Input: part model. Units: mm. Frame: model coordinates. Face numbers are marked on the shaded views. A direction names the side the tool comes from. Give positions to 0.01 mm unless a question says otherwise; leave off trailing zeros. Loops run counter-clockwise (first coordinate to the right, second up) from the corner with the lowest first, then second, coordinate; pieces in that order, holes last.
from build123d import *

# Parameters (mm, degrees)
F0_W     = 45
F0_H     = 44
F1_DEPTH = 23
F2_W     = 5
F2_H     = 5
F3_DEPTH = 5
F5_W     = 59
F5_H     = 23
F6_DEPTH = 2.75
F7_R     = 1


with BuildPart() as f1:
    # F0 (on Front) → F1 (new body)
    with BuildSketch(Plane.XZ):
        with Locations((22.5, 22)):
            Rectangle(F0_W, F0_H)
    extrude(amount=F1_DEPTH)

    # F2 (on face) → F3 (join)
    with BuildSketch(Plane.XY.offset(44)):
        with Locations((33, -11.5)):
            Rectangle(F2_W, F2_H)
    extrude(amount=F3_DEPTH)

    # F5 (on offset) → F6 (join)
    with BuildSketch(Plane.XY.offset(30)):
        with Locations((22.5, -11.5)):
            Rectangle(F5_W, F5_H)
    extrude(amount=F6_DEPTH)

    # F7
    f7_edges = [f1.edges().sort_by_distance(p)[0] for p in [
        (45, -11.5, 44),
        (22.5, 0, 44),
        (22.5, -23, 44),
        (0, -11.5, 44),
        (33, -9, 44),
        (35.5, -11.5, 44),
        (33, -14, 44),
        (30.5, -11.5, 44),
        (0, -11.5, 0),
        (45, -11.5, 0),
        (22.5, 0, 0),
        (22.5, -23, 0),
        (45, -23, 15),
        (45, 0, 15),
        (0, -23, 15),
        (0, -23, 38.375),
        (45, -23, 38.375),
        (45, 0, 38.375),
        (0, 0, 38.375),
        (0, 0, 15),
    ]]
    fillet(f7_edges, radius=F7_R)


solid = f1.part
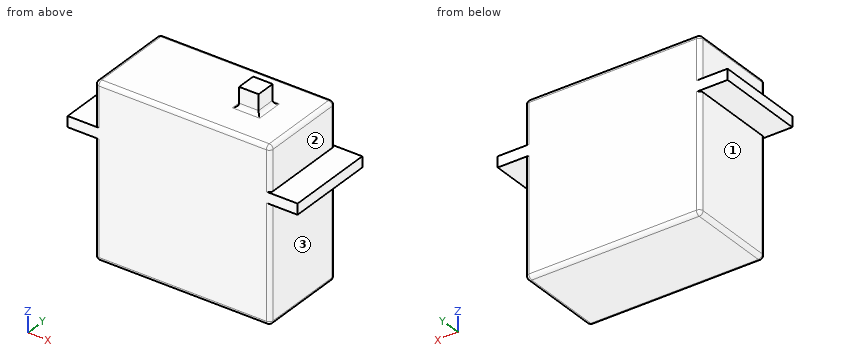
(1) Pin query (flat end, axial travel): pin 1 Ø4 at (x, y) = (-1.5, -12.5) entering from -Z; pin 2 Ø1.5 at (x, y) = (5, -20) entering from +Z; pin 3 Ø10 at (y, z) = (-4.5, 16.5) entering from -X. Return the tip coordinate at first contact, or that it passes through.
Values follow:
pin 1: stops at z = 0.13
pin 2: stops at z = 44
pin 3: stops at x = 0
(2) Cut plane B-B (x = 10). Return the cut outline in (y, z).
Values follow:
outline: (-23, 1) arc R1 ccw to (-22, 0) - (-1, 0) arc R1 ccw to (0, 1) - (0, 43) arc R1 ccw to (-1, 44) - (-22, 44) arc R1 ccw to (-23, 43) - close
(3) Ray query, probe 1 along Z at (x, y) = (24, -4.25); probe 2 along X at (y, z) = (-15.5, 37.5); probe 3 along Z at (x, y) = (47, -10.75). Return the intervals inside material, ascending.
Values follow:
probe 1: z = 0 to 44
probe 2: x = 0 to 45
probe 3: z = 30 to 32.75
(4) Reachability of the marked faces 1, 2 and 3 from +Z, -Z, +X, -X, +Y, -Y: full face, straight path, thin tool, end or side. Return the list, or none.
Values follow:
face 1: -Z, -X, +Y, -Y
face 2: +Z, +X, +Y, -Y
face 3: -Z, +X, +Y, -Y
(5) Cut plane D-D (y = -11.5). Return the cut outline in (x, z).
Values follow:
outline: (-7, 30) - (0, 30) - (0, 1) arc R1 ccw to (1, 0) - (44, 0) arc R1 ccw to (45, 1) - (45, 30) - (52, 30) - (52, 32.75) - (45, 32.75) - (45, 43) arc R1 ccw to (44, 44) - (36.5, 44) arc R1 cw to (35.5, 45) - (35.5, 49) - (30.5, 49) - (30.5, 45) arc R1 cw to (29.5, 44) - (1, 44) arc R1 ccw to (0, 43) - (0, 32.75) - (-7, 32.75) - close
(6) Cut plane A-A (z = 15). Return the cut outline in (x, y).
Values follow:
outline: (0, -22) arc R1 ccw to (1, -23) - (44, -23) arc R1 ccw to (45, -22) - (45, -1) arc R1 ccw to (44, 0) - (1, 0) arc R1 ccw to (0, -1) - close
(7) Cut plane C-C (y = -4.5). Return the cut outline in (x, z), and give its area (3 significant figures).
Values follow:
outline: (-7, 30) - (0, 30) - (0, 1) arc R1 ccw to (1, 0) - (44, 0) arc R1 ccw to (45, 1) - (45, 30) - (52, 30) - (52, 32.75) - (45, 32.75) - (45, 43) arc R1 ccw to (44, 44) - (1, 44) arc R1 ccw to (0, 43) - (0, 32.75) - (-7, 32.75) - close
area: 2,020 mm2
